Could you check a few things on this model? Use its own coordinates, in mm. Face numbers are marked on the shaded views. Coordinates: 2 decimals unless noted, no trailing zeros. Order: outer loops, then holes, each group sorted by start corner. A loop starts at its lowest first (then second) coordinate and runs counter-clockwise, first axis right, second up. Notation, with made-up numbers: (28.25, 7) -> (60.25, 7) arc R26 cw to (60.25, 42) -> close; hole circle Ø4 at (-38.5, -16.5). An arc over 180 degrees is marked (long way). Use a Markdown table: item, result. Add a question column.
1) If I drill on L1, parallel to Y at x = -17, z = 16; L2, parallel to Y at x = -15, z = 5.25; L3, parallel to Z at x = -4, y = -11, over which ranges is the centre line in solid material (lowest first)? Write a range as [from, to].
2) If we section it at B-B (z = 13.25): Give the number of separate pieces and of enclosed holes in the cut face, plus the area to 3 significant figures.
3) If we section it at C-C (y = 16.5): Write out the boundary of the cut face in (x, z), plus the area to 3 significant figures.
4) Thinking about a two-plate mould opening in Y: for the marked faces 1, 2 and 3, which applies, +Y half, -Y half, draft (parallel to the pull), parting line (faces both ways), or undercut?
5) Will these pins go through, and if not, where does the flat tip stop? pin 1 Ø1.5 at (x, y) = (-5.5, -2) entering from +Z; pin 2 Ø1 at (x, y) = (13.5, -8.5) entering from -Z; pin 3 Ø8 at (x, z) = (14.5, 9) entering from -Y; pin 4 Ø6 at (y, z) = (-19, 8) entering from -X.
6) If we section it at A-A (x = 0): Write out the boundary of the cut face in (y, z).
```python
from build123d import *

# Parameters (mm, degrees)
F0_R     = 1.5
F1_DEPTH = 17
F2_DEPTH = 2
F3_R     = 5


with BuildPart() as f1:
    # F0 (on Top) → F1 (new body)
    with BuildSketch(Plane.XY):
        with BuildLine():
            ThreePointArc((24.9419642857, 1.7024739558), (24.9854868588, 0.8517314298), (25, 0))
            ThreePointArc((25, 0), (24.9854868588, -0.8517314298), (24.9419642857, -1.7024739558))
            ThreePointArc((24.9419642857, -1.7024739558), (25.5347963833, -2.4845062142), (26.3214285714, -3.0712209232))
            ThreePointArc((26.3214285714, -3.0712209232), (26.4553194759, -1.538203962), (26.5, 0))
            ThreePointArc((26.5, 0), (26.4553194759, 1.538203962), (26.3214285714, 3.0712209232))
            ThreePointArc((26.3214285714, 3.0712209232), (25.5347963833, 2.4845062142), (24.9419642857, 1.7024739558))
        make_face()
        with BuildLine():
            ThreePointArc((-24.9419642857, 1.7024739558), (0, 25), (24.9419642857, 1.7024739558))
            ThreePointArc((24.9419642857, 1.7024739558), (25.5347963833, 2.4845062142), (26.3214285714, 3.0712209232))
            ThreePointArc((26.3214285714, 3.0712209232), (0, 26.5), (-26.3214285714, 3.0712209232))
            ThreePointArc((-26.3214285714, 3.0712209232), (-25.5347963833, 2.4845062142), (-24.9419642857, 1.7024739558))
        make_face()
        with BuildLine():
            ThreePointArc((26.3214285714, -3.0712209232), (25.5347963833, -2.4845062142), (24.9419642857, -1.7024739558))
            ThreePointArc((24.9419642857, -1.7024739558), (0, -25), (-24.9419642857, -1.7024739558))
            ThreePointArc((-24.9419642857, -1.7024739558), (-25.5347963833, -2.4845062142), (-26.3214285714, -3.0712209232))
            ThreePointArc((-26.3214285714, -3.0712209232), (0, -26.5), (26.3214285714, -3.0712209232))
        make_face()
        with BuildLine():
            ThreePointArc((-24.9419642857, -1.7024739558), (-25, 0), (-24.9419642857, 1.7024739558))
            ThreePointArc((-24.9419642857, 1.7024739558), (-25.5347963833, 2.4845062142), (-26.3214285714, 3.0712209232))
            ThreePointArc((-26.3214285714, 3.0712209232), (-26.4553194759, 1.538203962), (-26.5, 0))
            ThreePointArc((-26.5, 0), (-26.4553194759, -1.538203962), (-26.3214285714, -3.0712209232))
            ThreePointArc((-26.3214285714, -3.0712209232), (-25.5347963833, -2.4845062142), (-24.9419642857, -1.7024739558))
        make_face()
        with BuildLine():
            ThreePointArc((31.5, 0), (29.7853571071, 3.0103986447), (26.3214285714, 3.0712209232))
            ThreePointArc((26.3214285714, 3.0712209232), (26.4553194759, 1.538203962), (26.5, 0))
            ThreePointArc((26.5, 0), (26.4553194759, -1.538203962), (26.3214285714, -3.0712209232))
            ThreePointArc((26.3214285714, -3.0712209232), (29.7853571071, -3.0103986447), (31.5, 0))
        make_face()
        with BuildLine():
            ThreePointArc((29.5, 0), (28, -1.5), (26.5, 0))
            ThreePointArc((26.5, 0), (28, 1.5), (29.5, 0))
        make_face(mode=Mode.SUBTRACT)
        with BuildLine():
            ThreePointArc((-26.5, 0), (-26.4553194759, 1.538203962), (-26.3214285714, 3.0712209232))
            ThreePointArc((-26.3214285714, 3.0712209232), (-31.5, 0), (-26.3214285714, -3.0712209232))
            ThreePointArc((-26.3214285714, -3.0712209232), (-26.4553194759, -1.538203962), (-26.5, 0))
        make_face()
        with Locations((-28, 0)):
            Circle(F0_R, mode=Mode.SUBTRACT)
    extrude(amount=F1_DEPTH)

    # F0 (on Top) → F2 (join)
    with BuildSketch(Plane.XY):
        with BuildLine():
            ThreePointArc((24.9419642857, 1.7024739558), (24.9854868588, 0.8517314298), (25, 0))
            ThreePointArc((25, 0), (24.9854868588, -0.8517314298), (24.9419642857, -1.7024739558))
            ThreePointArc((24.9419642857, -1.7024739558), (25.5347963833, -2.4845062142), (26.3214285714, -3.0712209232))
            ThreePointArc((26.3214285714, -3.0712209232), (26.4553194759, -1.538203962), (26.5, 0))
            ThreePointArc((26.5, 0), (26.4553194759, 1.538203962), (26.3214285714, 3.0712209232))
            ThreePointArc((26.3214285714, 3.0712209232), (25.5347963833, 2.4845062142), (24.9419642857, 1.7024739558))
        make_face()
        with BuildLine():
            ThreePointArc((-24.9419642857, 1.7024739558), (0, 25), (24.9419642857, 1.7024739558))
            ThreePointArc((24.9419642857, 1.7024739558), (25.5347963833, 2.4845062142), (26.3214285714, 3.0712209232))
            ThreePointArc((26.3214285714, 3.0712209232), (0, 26.5), (-26.3214285714, 3.0712209232))
            ThreePointArc((-26.3214285714, 3.0712209232), (-25.5347963833, 2.4845062142), (-24.9419642857, 1.7024739558))
        make_face()
        with BuildLine():
            ThreePointArc((26.3214285714, -3.0712209232), (25.5347963833, -2.4845062142), (24.9419642857, -1.7024739558))
            ThreePointArc((24.9419642857, -1.7024739558), (0, -25), (-24.9419642857, -1.7024739558))
            ThreePointArc((-24.9419642857, -1.7024739558), (-25.5347963833, -2.4845062142), (-26.3214285714, -3.0712209232))
            ThreePointArc((-26.3214285714, -3.0712209232), (0, -26.5), (26.3214285714, -3.0712209232))
        make_face()
        with BuildLine():
            ThreePointArc((-24.9419642857, -1.7024739558), (-25, 0), (-24.9419642857, 1.7024739558))
            ThreePointArc((-24.9419642857, 1.7024739558), (-25.5347963833, 2.4845062142), (-26.3214285714, 3.0712209232))
            ThreePointArc((-26.3214285714, 3.0712209232), (-26.4553194759, 1.538203962), (-26.5, 0))
            ThreePointArc((-26.5, 0), (-26.4553194759, -1.538203962), (-26.3214285714, -3.0712209232))
            ThreePointArc((-26.3214285714, -3.0712209232), (-25.5347963833, -2.4845062142), (-24.9419642857, -1.7024739558))
        make_face()
        with BuildLine():
            ThreePointArc((31.5, 0), (29.7853571071, 3.0103986447), (26.3214285714, 3.0712209232))
            ThreePointArc((26.3214285714, 3.0712209232), (26.4553194759, 1.538203962), (26.5, 0))
            ThreePointArc((26.5, 0), (26.4553194759, -1.538203962), (26.3214285714, -3.0712209232))
            ThreePointArc((26.3214285714, -3.0712209232), (29.7853571071, -3.0103986447), (31.5, 0))
        make_face()
        with BuildLine():
            ThreePointArc((29.5, 0), (28, -1.5), (26.5, 0))
            ThreePointArc((26.5, 0), (28, 1.5), (29.5, 0))
        make_face(mode=Mode.SUBTRACT)
        with BuildLine():
            ThreePointArc((-26.5, 0), (-26.4553194759, 1.538203962), (-26.3214285714, 3.0712209232))
            ThreePointArc((-26.3214285714, 3.0712209232), (-31.5, 0), (-26.3214285714, -3.0712209232))
            ThreePointArc((-26.3214285714, -3.0712209232), (-26.4553194759, -1.538203962), (-26.5, 0))
        make_face()
        with Locations((-28, 0)):
            Circle(F0_R, mode=Mode.SUBTRACT)
        with BuildLine():
            ThreePointArc((24.9419642857, -1.7024739558), (24.5, 0), (24.9419642857, 1.7024739558))
            ThreePointArc((24.9419642857, 1.7024739558), (0, 25), (-24.9419642857, 1.7024739558))
            ThreePointArc((-24.9419642857, 1.7024739558), (-24.6122924418, 0.879452955), (-24.5, 0))
            ThreePointArc((-24.5, 0), (-24.6122924418, -0.879452955), (-24.9419642857, -1.7024739558))
            ThreePointArc((-24.9419642857, -1.7024739558), (0, -25), (24.9419642857, -1.7024739558))
        make_face()
        with BuildLine():
            ThreePointArc((-24.5, 0), (-24.6122924418, 0.879452955), (-24.9419642857, 1.7024739558))
            ThreePointArc((-24.9419642857, 1.7024739558), (-25, 0), (-24.9419642857, -1.7024739558))
            ThreePointArc((-24.9419642857, -1.7024739558), (-24.6122924418, -0.879452955), (-24.5, 0))
        make_face()
        with BuildLine():
            ThreePointArc((24.9419642857, -1.7024739558), (24.9854868588, -0.8517314298), (25, 0))
            ThreePointArc((25, 0), (24.9854868588, 0.8517314298), (24.9419642857, 1.7024739558))
            ThreePointArc((24.9419642857, 1.7024739558), (24.5, 0), (24.9419642857, -1.7024739558))
        make_face()
        with Locations((-28, 0)):
            Circle(F0_R)
        with BuildLine():
            ThreePointArc((29.5, 0), (28, 1.5), (26.5, 0))
            ThreePointArc((26.5, 0), (28, -1.5), (29.5, 0))
        make_face()
    extrude(amount=F2_DEPTH)

    # F3
    f3_edges = [f1.edges().sort_by_distance(p)[0] for p in [
        (-26.321429, 3.071221, 8.5),
        (-26.321429, -3.071221, 8.5),
        (26.321429, -3.071221, 8.5),
        (26.321429, 3.071221, 8.5),
    ]]
    fillet(f3_edges, radius=F3_R)


solid = f1.part
```
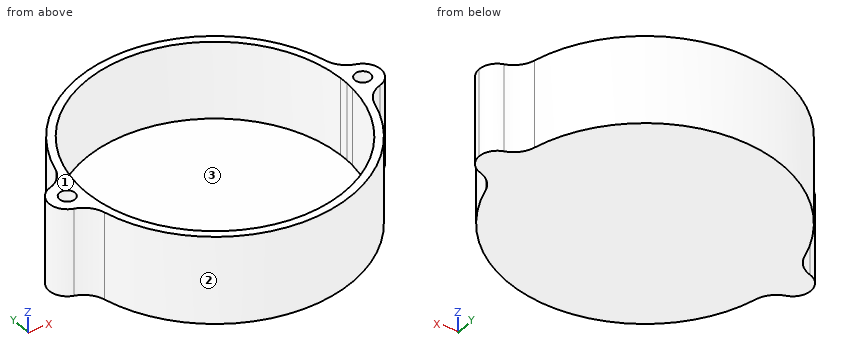
Answer sheet:
| question | item | result |
|---|---|---|
| 1 | L1 | [-20.33, -18.33], [18.33, 20.33] |
| 1 | L2 | [-21.85, -20], [20, 21.85] |
| 1 | L3 | [0, 2] |
| 2 | separate pieces | 1 |
| 2 | enclosed holes | 3 |
| 2 | area | 298 mm2 |
| 3 | outline | (-20.74, 0) -> (20.74, 0) -> (20.74, 17) -> (18.78, 17) -> (18.78, 2) -> (-18.78, 2) -> (-18.78, 17) -> (-20.74, 17) -> close |
| 3 | area | 142 mm2 |
| 4 | face 1 | draft |
| 4 | face 2 | -Y half |
| 4 | face 3 | undercut |
| 5 | pin 1 | z = 2 |
| 5 | pin 2 | z = 0 |
| 5 | pin 3 | y = -24.33 |
| 5 | pin 4 | x = -21.12 |
| 6 | outline | (-26.5, 0) -> (26.5, 0) -> (26.5, 17) -> (25, 17) -> (25, 2) -> (-25, 2) -> (-25, 17) -> (-26.5, 17) -> close |
